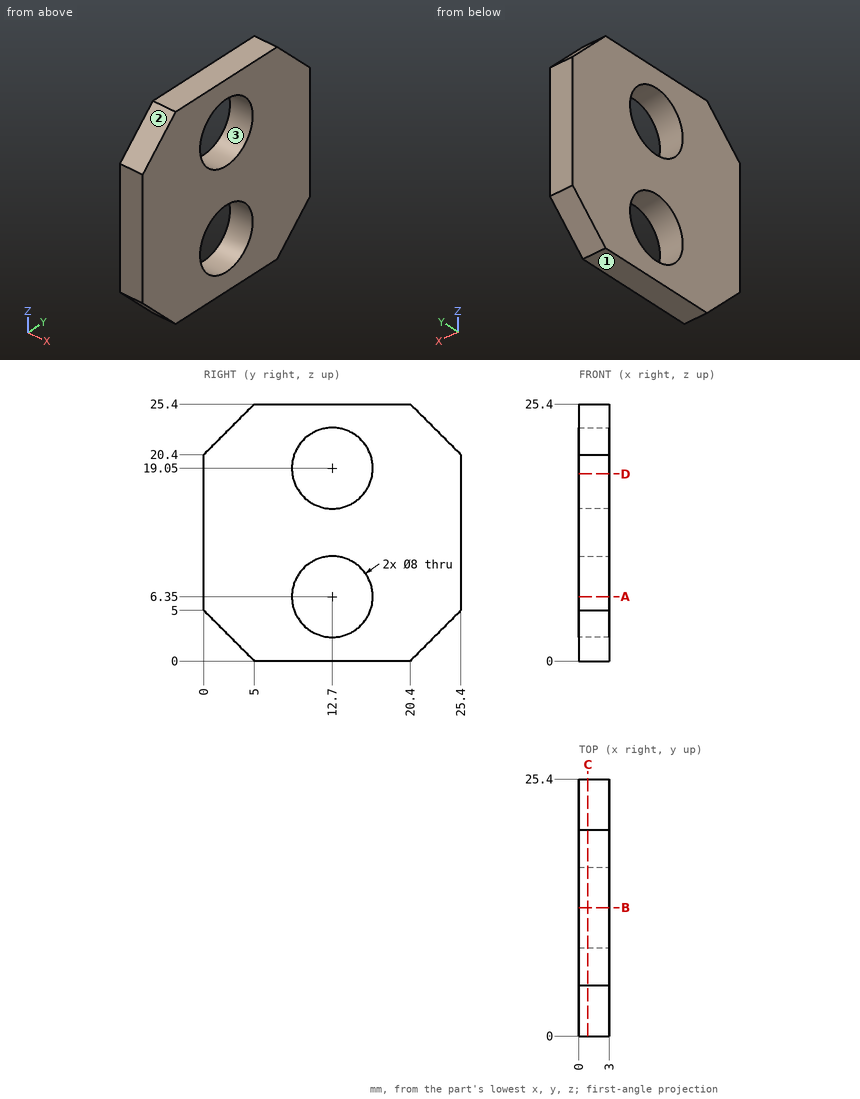
Part print with two shaded views. Sizes in mm from the minimum x, y, z corner. Round coordinates to 2 decimals unless told otherwise and drop trailing zeros. Loops run counter-clockwise (first coordinate to the right, second up) from the corner with the lowest first, then second, coordinate; pieces in that order, holes last. Notation, with made-up numbers: (7, 84.5) - (15, 84.5) arc R9 ccw to (15, 95.5) - close; hole circle Ø8 at (85.25, 82). An arc over 180 degrees is marked (long way). Answer as a JSON object with one key per item and string values.
Item 1: Band-saw the part on C-C on x = 0.9. List the corners of the cut face in (y, z), plus the area to 3 significant figures.
Output:
{"outline": "(0, 5) - (5, 0) - (20.4, 0) - (25.4, 5) - (25.4, 20.4) - (20.4, 25.4) - (5, 25.4) - (0, 20.4) - close; hole circle Ø8 at (12.7, 6.35); hole circle Ø8 at (12.7, 19.05)", "area": "495 mm2"}
Item 2: Pin check, flat tip, straight feed: pin 1 (1 mm diameter, centred on x = 1.5, z = 21.5, fed in from +Y). Stop position of the tip, or through.
Output:
{"pin 1": "y = 24.8"}
Item 3: Pull direction Z, two halves, no side cores. Call the marked faces 1, 2 and 3: pulls with the +Z half, pulls with the -Z half, needs draft (parallel to the pull), parting line crosses it, or undercut.
Output:
{"face 1": "pulls with the -Z half", "face 2": "pulls with the +Z half", "face 3": "undercut"}
Item 4: Wall check: L1, parallel to Y at x = 1.05, z = 6.35; L2, parallel to Z at x = 0.4, y = 9.5; L3, parallel to Y at x = 1.1, z = 22.25. Give the ranges that are in metal, low to high.
Output:
{"L1": "0 to 8.7, 16.7 to 25.4", "L2": "0 to 3.95, 8.75 to 16.65, 21.45 to 25.4", "L3": "1.85 to 10.3, 15.1 to 23.55"}
Item 5: Band-saw the part on B-B on y = 12.7. List the corners of the cut face in (x, z).
Output:
{"outline": "(0, 0) - (3, 0) - (3, 2.35) - (0, 2.35) - close; (0, 10.35) - (3, 10.35) - (3, 15.05) - (0, 15.05) - close; (0, 23.05) - (3, 23.05) - (3, 25.4) - (0, 25.4) - close"}
Item 6: Band-saw the part on D-D on z = 18.5. List the corners of the cut face in (x, y).
Output:
{"outline": "(0, 0) - (3, 0) - (3, 8.74) - (0, 8.74) - close; (0, 16.66) - (3, 16.66) - (3, 25.4) - (0, 25.4) - close"}
Item 7: Band-saw the part on A-A on z = 6.35. List the corners of the cut face in (x, y).
Output:
{"outline": "(0, 0) - (3, 0) - (3, 8.7) - (0, 8.7) - close; (0, 16.7) - (3, 16.7) - (3, 25.4) - (0, 25.4) - close"}
